Input: part model. Units: mm. Frame: model coordinates. A direction names the side the tool comes from. Round coordinates to 2 decimals unless told otherwise and drop trailing zeros. Write each loop counter-clockwise with the first axis right and the second up, starting at its lowest first coordinate (ties: lowest second). Pieces come first, ordered by that corner, then holes. Notation, with made-up numbers: (42, 1) -> (62, 1) arc R25 cw to (62, 24) -> close; hole circle Ø1 at (47.25, 89). An arc over 180 degrees is marked (long way). Write item = value, one per line.
```python
from build123d import *

# Parameters (mm, degrees)
BOSS_EXTRU_1_DEPTH           = 100
ESQUISSE2_W                  = 6
ESQUISSE2_H                  = 6.000000000000014
ESQUISSE2_H_2                = 6.000000000000005
BOSS_EXTRU_2_DEPTH           = 3
ESQUISSE3_R                  = 2.2500000000000027
ESQUISSE3_R_2                = 2.250000000000001
ENL_V_MAT_EXTRU_1_DEPTH      = 5
ENL_V_MAT_EXTRU_2_DEPTH      = 106.73176853427184
ENL_V_MAT_EXTRU_2_DEPTH_BACK = 106.73176853427184
ESQUISSE4_R                  = 1.7500000000000013
ESQUISSE4_R_2                = 1.75
CONG_1_R                     = 2
ENL_V_MAT_EXTRU_3_DEPTH      = 6
CONG_2_R                     = 4
ENL_V_MAT_EXTRU_5_DEPTH      = 6.000001
CONG_3_R                     = 4
ESQUISSE7_R                  = 2.2500000000000027
ESQUISSE7_R_2                = 2.250000000000002
ENL_V_MAT_EXTRU_6_DEPTH      = 6


with BuildPart() as part:
    # Esquisse1 → Boss.-Extru.1 (new body)
    with BuildSketch(Plane.XY):
        Polygon((0, 0), (0, 34.167556264006286), (-26.019007623520746, 12.33501656351095), (-29.875733281640006, 16.9312832222248), (0, 42), (5.999999999999995, 42), (6, 2.4e-16), align=None)
    extrude(amount=BOSS_EXTRU_1_DEPTH)

    # Esquisse2 → Boss.-Extru.2 (add)
    with BuildSketch(Plane(origin=(-20.680962813256418, 24.64661173100532, 0), x_dir=(0.7660444431189743, 0.6427876096865438, 0), z_dir=(-0.6427876096865438, 0.7660444431189745, 0))):
        with Locations((-9.002920393165164, -97)):
            Rectangle(ESQUISSE2_W, ESQUISSE2_H)
        with Locations((-9.002920393165164, -3.0000000000000027)):
            Rectangle(ESQUISSE2_W, ESQUISSE2_H_2)
    extrude(amount=BOSS_EXTRU_2_DEPTH)

    # Esquisse3 → Enlèv. mat.-Extru.1 (cut)
    with BuildSketch(Plane(origin=(-22.609325642316065, 26.94474506036225, 0), x_dir=(0.7660444431189746, 0.6427876096865436, 0), z_dir=(-0.6427876096865435, 0.7660444431189745, 0))):
        with Locations(Location((-9.002920393165152, -97, 0), (0, 0, 180))):
            Circle(ESQUISSE3_R)
        with Locations(Location((-9.002920393165152, -3.0000000000000027, 0), (0, 0, 180))):
            Circle(ESQUISSE3_R_2)
    extrude(amount=-ENL_V_MAT_EXTRU_1_DEPTH, mode=Mode.SUBTRACT)

    # Esquisse4 → Enlèv. mat.-Extru.2 (cut, two sides: drawn at the far end of the back side and taken through both)
    with BuildSketch(Plane(origin=(-19.395387593883342, 23.114522844767386, 0), x_dir=(0.7660444431189743, 0.6427876096865437, 0), z_dir=(-0.6427876096865437, 0.7660444431189743, 0)).offset(-ENL_V_MAT_EXTRU_2_DEPTH_BACK)):
        with Locations(Location((-9.002920393165155, -97, 0), (0, 0, 180))):
            Circle(ESQUISSE4_R)
        with Locations(Location((-9.002920393165155, -3.0000000000000027, 0), (0, 0, 180))):
            Circle(ESQUISSE4_R_2)
    extrude(amount=ENL_V_MAT_EXTRU_2_DEPTH + ENL_V_MAT_EXTRU_2_DEPTH_BACK, mode=Mode.SUBTRACT)

    # Congé1
    cong_1_edges = [part.edges().sort_by_distance(p)[0] for p in [
        (-28.91155186711019, 15.782216557546342, 100),
        (-30.83991469616982, 18.080349886903274, 94),
        (-26.243648037455976, 21.937075545022537, 100),
        (-26.243648037455976, 21.937075545022537, 94),
        (-26.243648037455976, 21.937075545022537, 0),
        (-30.83991469616982, 18.080349886903274, 6.000000000000005),
        (-26.243648037455976, 21.937075545022537, 6.000000000000005),
        (-28.91155186711019, 15.782216557546342, 0),
    ]]
    fillet(cong_1_edges, radius=CONG_1_R)

    # Esquisse5 → Enlèv. mat.-Extru.3 (cut)
    with BuildSketch(Plane(origin=(6, 7.4e-16, 0), x_dir=(0, 0, -1), z_dir=(1, 1.2e-16, 0))):
        Polygon((-100, -4.5e-16), (-73.00000000000001, 0), (-73.00000000000001, 34.167556264006286), (-100, 34.167556264006286), align=None)
        Polygon((0, 0), (-51, -6.25e-15), (-51, 34.167556264006286), (0, 34.167556264006286), align=None)
    extrude(amount=-ENL_V_MAT_EXTRU_3_DEPTH, mode=Mode.SUBTRACT)

    # Congé2
    cong_2_edges = [part.edges().sort_by_distance(p)[0] for p in [
        (0, 34.167556264006286, 62.00000000000001),
    ]]
    fillet(cong_2_edges, radius=CONG_2_R)

    # Esquisse6 → Enlèv. mat.-Extru.5 (cut)
    with BuildSketch(Plane(origin=(-20.68096281325642, 24.646611731005315, 0), x_dir=(0.7660444431189746, 0.6427876096865437, 0), z_dir=(-0.6427876096865437, 0.7660444431189746, 0))):
        Polygon((-8.002920393165189, -8.000000000000007), (11.997079606834813, -8.000000000000007), (11.997079606834824, -92), (-8.002920393165178, -92), align=None)
    extrude(amount=-ENL_V_MAT_EXTRU_5_DEPTH, mode=Mode.SUBTRACT)

    # Congé3
    cong_3_edges = [part.edges().sort_by_distance(p)[0] for p in [
        (0, 34.167556264006286, 86.5),
        (0, 42, 50),
        (5.999999999999996, 38.08377813200315, 100),
        (2.9999999999999964, 34.167556264006286, 73.00000000000001),
        (3, 4e-16, 73.00000000000001),
        (5.999999999999996, 38.08377813200315, 0),
        (3, -5.85e-15, 51),
        (0, 34.167556264006286, 25.5),
        (2.9999999999999964, 34.167556264006286, 51),
        (-24.88319268010449, 17.204300331614043, 92),
        (-24.8831926801045, 17.20430033161404, 8.000000000000007),
        (-9.562303817725006, 30.060052525344915, 8.000000000000007),
        (-9.562303817724995, 30.060052525344922, 92),
    ]]
    fillet(cong_3_edges, radius=CONG_3_R)

    # Esquisse7 → Enlèv. mat.-Extru.6 (cut)
    with BuildSketch(Plane(origin=(6, 7.4e-16, 0), x_dir=(0, 0, -1), z_dir=(1, 1.3e-16, 0))):
        with Locations(Location((-62, 22, 0), (0, 0, 90))):
            Circle(ESQUISSE7_R)
        with Locations(Location((-62, 6, 0), (0, 0, 90))):
            Circle(ESQUISSE7_R_2)
    extrude(amount=-ENL_V_MAT_EXTRU_6_DEPTH, mode=Mode.SUBTRACT)


solid = part.part
```
1) Cut plane D-D (z = 62). Return the cut outline in (x, y).
Solutions:
outline = (-29.88, 16.93) -> (-26.02, 12.34) -> (-22.95, 14.91) -> (-26.81, 19.5) -> close; (-11.49, 32.36) -> (-7.63, 27.76) -> (-6.57, 28.65) arc R4 cw to (0, 25.59) -> (0, 24.25) -> (6, 24.25) -> (6, 42) -> (1.46, 42) arc R4 ccw to (-1.12, 41.06) -> close; (0, 0) -> (6, 0) -> (6, 3.75) -> (0, 3.75) -> close; (0, 8.25) -> (6, 8.25) -> (6, 19.75) -> (0, 19.75) -> close
2) Cut plane B-B (z = 17.5). Return the cut outline in (x, y), and give its area (3 significant figures).
Solutions:
outline = (-29.88, 16.93) -> (-26.02, 12.34) -> (-22.95, 14.91) -> (-26.81, 19.5) -> close; (-11.49, 32.36) -> (-7.63, 27.76) -> (-1.12, 33.23) arc R4 cw to (1.46, 34.17) -> (6, 34.17) -> (6, 42) -> (1.46, 42) arc R4 ccw to (-1.12, 41.06) -> close
area = 146 mm^2
3) Access query for faces 1 (the face through (-30.417, 18.463, 94.601)), 2 (the face through (-9.59, 30.09, 49.47)), 3 (the face through (-17, 24, 92)). Directions: +Z, -Z, +X, -X, +Y, -Y. A direction counts if a zero-diameter tool reaches every point of the face in a straight line with its end or side. Return the directions, or none.
Solutions:
face_1 = -X
face_2 = -X, -Y
face_3 = none
4) Cut plane C-C (x = -16). Return the cut outline in (y, z).
Solutions:
outline = (20.74, 0) -> (28.57, 0) -> (28.57, 8) -> (20.74, 8) -> close; (20.74, 92) -> (28.57, 92) -> (28.57, 100) -> (20.74, 100) -> close
5) First-contact query: P1, Ø7, axis at y = 6, z = 62, coming from the -X side; P2, Ø1.5, axis at x = -26.5, z = 36.5, coming from the +Y side; P3, Ø5, axis at x = 2.5, z = 84.5, coming from the -Y side. Flat tips, straight axial feed; report the tip coordinate or a pass-through.
Solutions:
P1 = 0
P2 = 19.5
P3 = 33.89
6) Line query: L1, parallel to Z at x = 3.4, y = 6; L2, parallel to Z at x = -18, y = 22.5; L3, parallel to X at y = 29, z = 58.5. Output: solid intervals per line, ascending. Write a range as from..to.
Solutions:
L1 = 51..59.75, 64.25..73
L2 = 0..8, 92..100
L3 = -8.67..-6.09, -1.91..6
7) Cut plane A-A (y = 6). Return the cut outline in (x, z), and give its area (3 significant figures).
Solutions:
outline = (0, 51) -> (6, 51) -> (6, 59.75) -> (0, 59.75) -> close; (0, 64.25) -> (6, 64.25) -> (6, 73) -> (0, 73) -> close
area = 105 mm^2
8) Draft query along Z for faces 4 (the face through (3, 0, 62)), 5 (the face through (-28.43, 16.1, 0.6)), 6 (the face through (-10.41, 29.29, 90.8)). Return one class per face: +Z half, -Z half, draft (parallel to the pull), parting line (faces both ways), or undercut.
Solutions:
face_4 = draft
face_5 = -Z half
face_6 = undercut
